The listing builds one solid part. Answer for the finished solid, in the listing's coordinates (mm). A direction names the side the tool comes from. Round coordinates to 2 decimals unless told otherwise and drop trailing zeros. Loops run counter-clockwise (first coordinate to the right, second up) from the corner with the lowest first, then second, coordinate; pieces in that order, holes last. Notation, with made-up numbers: (69, 85.5) - (80, 85.5) arc R19 ccw to (80, 93.5) - close; hole circle Ø11 at (54.25, 5.5). An arc over 180 degrees is marked (long way). One line per item, written item: value.
```python
from build123d import *

# Parameters (mm, degrees)
CROQUIS1_W              = 110
CROQUIS1_H              = 90
SALIENTE_EXTRUIR1_DEPTH = 2
CROQUIS3_R              = 3
SALIENTE_EXTRUIR2_DEPTH = 5
CROQUIS4_R              = 1.5
CORTAR_EXTRUIR1_DEPTH   = 4
CROQUIS5_W              = 3
CROQUIS5_H              = 25
SALIENTE_EXTRUIR3_DEPTH = 13
CROQUIS6_W              = 3
CROQUIS6_H              = 37
CROQUIS6_H_2            = 15
CROQUIS6_H_3            = 12
SALIENTE_EXTRUIR4_DEPTH = 3
CROQUIS7_W              = 106
CROQUIS7_H              = 86
CROQUIS7_W_2            = 104
CROQUIS7_H_2            = 84
CORTAR_EXTRUIR2_DEPTH   = 5
CORTAR_EXTRUIR3_DEPTH   = 12
CROQUIS9_R              = 1.6
CORTAR_EXTRUIR4_DEPTH   = 12
CORTAR_EXTRUIR5_DEPTH   = 12


with BuildPart() as part:
    # Croquis1 → Saliente-Extruir1 (new body)
    with BuildSketch(Plane(origin=(0, 0, 0), x_dir=(1, 0, 0), z_dir=(0, 1, 0))):
        Rectangle(CROQUIS1_W, CROQUIS1_H)
    extrude(amount=SALIENTE_EXTRUIR1_DEPTH)

    # Croquis3 → Saliente-Extruir2 (add)
    with BuildSketch(Plane(origin=(0, 2, 0), x_dir=(1, 0, 0), z_dir=(0, 1, 0))):
        with Locations(Location((-47.19, -37.19, 0), (0, 0, 90))):
            Circle(CROQUIS3_R)
        with Locations(Location((-47.19, 37.19, 0), (0, 0, 90))):
            Circle(CROQUIS3_R)
        with Locations(Location((35.36, -37.19, 0), (0, 0, 90))):
            Circle(CROQUIS3_R)
        with Locations(Location((35.36, 37.19, 0), (0, 0, 90))):
            Circle(CROQUIS3_R)
    extrude(amount=SALIENTE_EXTRUIR2_DEPTH)

    # Croquis4 → Cortar-Extruir1 (cut)
    with BuildSketch(Plane(origin=(0, 7, 0), x_dir=(1, 0, 0), z_dir=(0, 1, 0))):
        with Locations(Location((-47.19, -37.19, 0), (0, 0, 270))):
            Circle(CROQUIS4_R)
        with Locations(Location((35.36, -37.19, 0), (0, 0, 270))):
            Circle(CROQUIS4_R)
        with Locations(Location((35.36, 37.19, 0), (0, 0, 270))):
            Circle(CROQUIS4_R)
        with Locations(Location((-47.19, 37.19, 0), (0, 0, 270))):
            Circle(CROQUIS4_R)
    extrude(amount=-CORTAR_EXTRUIR1_DEPTH, mode=Mode.SUBTRACT)

    # Croquis5 → Saliente-Extruir3 (add)
    with BuildSketch(Plane(origin=(0, 2, 0), x_dir=(1, 0, 0), z_dir=(0, 1, 0))):
        Polygon((52, -39), (55, -39), (55, -45), (-55, -45), (-55, -18), (-52, -18), (-52, -42), (52, -42), align=None)
        Polygon((-55, 45), (55, 45), (55, 13), (52, 13), (52, 42), (-52, 42), (-52, 19), (-55, 19), align=None)
        with Locations((53.5, -14.5)):
            Rectangle(CROQUIS5_W, CROQUIS5_H)
    extrude(amount=SALIENTE_EXTRUIR3_DEPTH)

    # Croquis6 → Saliente-Extruir4 (add)
    with BuildSketch(Plane(origin=(0, 2, 0), x_dir=(1, 0, 0), z_dir=(0, 1, 0))):
        with Locations((-53.5, 0.5)):
            Rectangle(CROQUIS6_W, CROQUIS6_H)
        with Locations((53.5, 5.5)):
            Rectangle(CROQUIS6_W, CROQUIS6_H_2)
        with Locations((53.5, -33)):
            Rectangle(CROQUIS6_W, CROQUIS6_H_3)
    extrude(amount=SALIENTE_EXTRUIR4_DEPTH)

    # Croquis7 → Cortar-Extruir2 (cut)
    with BuildSketch(Plane(origin=(0, 15, 0), x_dir=(1, 0, 0), z_dir=(0, 1, 0))):
        Rectangle(CROQUIS7_W, CROQUIS7_H)
        Rectangle(CROQUIS7_W_2, CROQUIS7_H_2, mode=Mode.SUBTRACT)
    extrude(amount=-CORTAR_EXTRUIR2_DEPTH, mode=Mode.SUBTRACT)

    # Croquis8 → Cortar-Extruir3 (cut)
    with BuildSketch(Plane(origin=(0, 15, 0), x_dir=(1, 0, 0), z_dir=(0, 1, 0))):
        Polygon((55, -10.5), (54, -9.5), (54, -12.5), (55, -11.5), align=None)
        Polygon((55, 22.5), (55, 21.5), (54, 20.5), (54, 23.5), align=None)
    extrude(amount=-CORTAR_EXTRUIR3_DEPTH, mode=Mode.SUBTRACT)

    # Croquis9 → Cortar-Extruir4 (cut)
    with BuildSketch(Plane(origin=(55, 0, 0), x_dir=(0, 0, -1), z_dir=(1, 0, 0))):
        with Locations((-6.25, 12)):
            Circle(CROQUIS9_R)
        with Locations((17.25, 12)):
            Circle(CROQUIS9_R)
    extrude(amount=-CORTAR_EXTRUIR4_DEPTH, mode=Mode.SUBTRACT)

    # Croquis11 → Cortar-Extruir5 (cut)
    with BuildSketch(Plane(origin=(0, 15, 0), x_dir=(1, 0, 0), z_dir=(0, 1, 0))):
        Polygon((-55, -23.5), (-54, -22.5), (-54, -25.5), (-55, -24.5), align=None)
        Polygon((-55, 25.5), (-55, 24.5), (-54, 23.5), (-54, 26.5), align=None)
    extrude(amount=-CORTAR_EXTRUIR5_DEPTH, mode=Mode.SUBTRACT)


solid = part.part
```
1) For faces 4 (the cylindrical face through (54, 13, -16)), 5 (the flat face through (54, 10, 27)), 6 (the cylindrical face through (34.45, 5.03, -38.38)), 7 (the flat face through (-54, 5, -1)), determine the directions among +Z, -Z, +X, -X, +Y, -Y from which every point of the face is accessible in a straight line to the end or side of a thin tool.
Final values:
face 4: +X, -X
face 5: +X, +Y
face 6: +Y
face 7: -X, +Y
2) For a pull along X with two mould halves and no side action, classify faces 1 (the flat face through (-1, 7, -45)), 2 (the cylindrical face through (37.185, 4.465, -34.809)), 3 (the flat face through (55, 4, -1)) as released by +X, released by -X, zero draft, split by the parting line, or undercut.
Final values:
face 1: zero draft
face 2: undercut
face 3: released by +X
3) A cutting plane is placed at D-D on z = 37.19. Give the vertices of the cut face in (x, y), and give its area (3 significant figures).
Final values:
outline: (-55, 0) - (55, 0) - (55, 5) - (52, 5) - (52, 2) - (38.36, 2) - (38.36, 7) - (36.86, 7) - (36.86, 3) - (33.86, 3) - (33.86, 7) - (32.36, 7) - (32.36, 2) - (-44.19, 2) - (-44.19, 7) - (-45.69, 7) - (-45.69, 3) - (-48.69, 3) - (-48.69, 7) - (-50.19, 7) - (-50.19, 2) - (-52, 2) - (-52, 10) - (-53, 10) - (-53, 15) - (-55, 15) - close
area: 299 mm2
4) A cutting plane is placed at A-A on z = 6.25. Give the vertices of the cut face in (x, y).
Final values:
outline: (-55, 0) - (55, 0) - (55, 10.4) - (53, 10.4) - (53, 10) - (52, 10) - (52, 2) - (-52, 2) - (-52, 5) - (-55, 5) - close; (53, 13.6) - (55, 13.6) - (55, 15) - (53, 15) - close
5) A cutting plane is placed at C-C on z = -37.19. Give the vertices of the cut face in (x, y).
Final values:
outline: (-55, 0) - (55, 0) - (55, 15) - (53, 15) - (53, 10) - (52, 10) - (52, 2) - (38.36, 2) - (38.36, 7) - (36.86, 7) - (36.86, 3) - (33.86, 3) - (33.86, 7) - (32.36, 7) - (32.36, 2) - (-44.19, 2) - (-44.19, 7) - (-45.69, 7) - (-45.69, 3) - (-48.69, 3) - (-48.69, 7) - (-50.19, 7) - (-50.19, 2) - (-52, 2) - (-52, 10) - (-53, 10) - (-53, 15) - (-55, 15) - close
6) Consider L1, parallel to X at y = 5.45, z = -37.19; L2, parallel to Z at x = -44.5, y = 13.25; L3, parallel to Y at x = 53.6, z = -17.25. Determine where each line is inside the solid, lowest interval first.
Final values:
L1: -55 to -52, -50.19 to -48.69, -45.69 to -44.19, 32.36 to 33.86, 36.86 to 38.36, 52 to 55
L2: -45 to -43, 43 to 45
L3: 0 to 10.4, 13.6 to 15
7) Each of these flat-tipped pins is pushed along its axis until it touches: pin 1 Ø5 at (x, z) = (2, -33.5) entering from +Y; pin 2 Ø0.9 at (x, z) = (54, 30.5) entering from +Y; pin 3 Ø2.5 at (y, z) = (7, -2) entering from +X; pin 4 Ø0.9 at (y, z) = (11.5, -22) entering from +X. Where does it stop, or does it pass through?
Final values:
pin 1: y = 2
pin 2: y = 5
pin 3: through
pin 4: x = 54
8) A cutting plane is placed at B-B on x = -14. Give the vertices of the cut face in (y, z).
Final values:
outline: (0, -45) - (15, -45) - (15, -43) - (10, -43) - (10, -42) - (2, -42) - (2, 42) - (10, 42) - (10, 43) - (15, 43) - (15, 45) - (0, 45) - close
